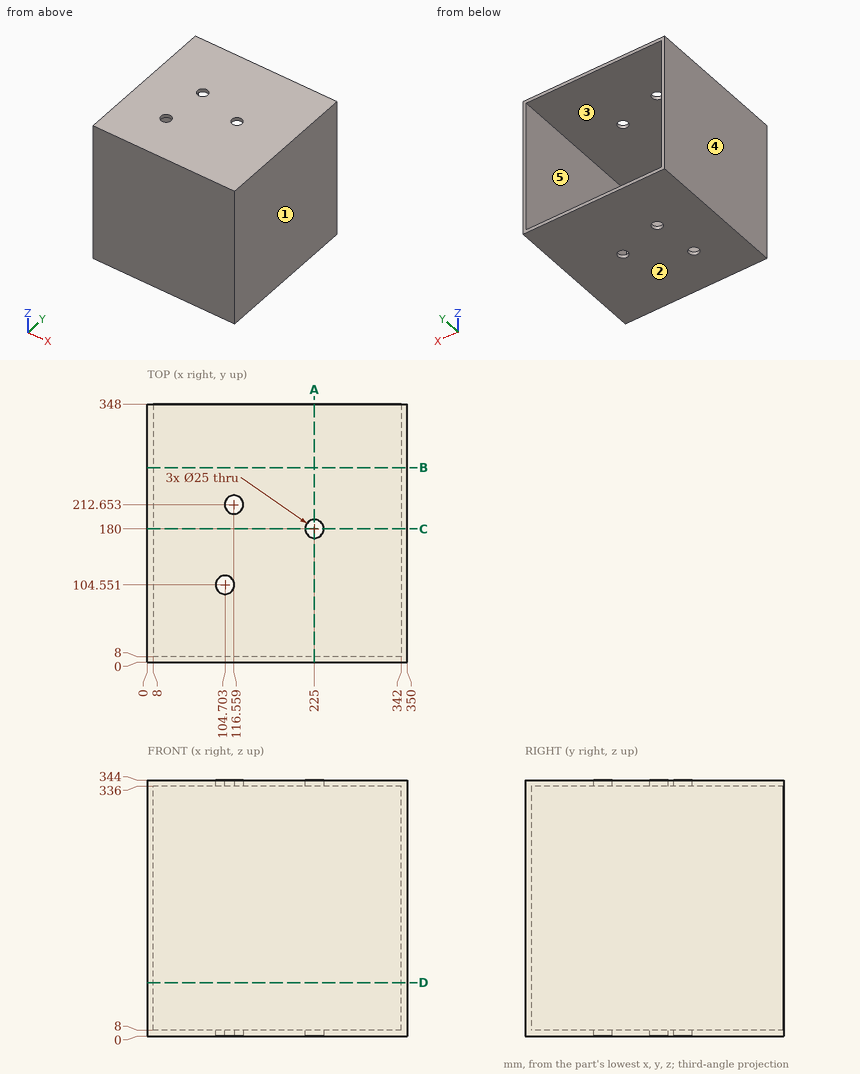
Verification items for this drawing (mm, ordinates from the low corner). A direction names the side the tool comes from. Round coordinates to 2 decimals unless told otherwise and drop trailing zeros. Loops run counter-clockwise (first coordinate to the right, second up) from the corner with the lowest first, then second, coordinate; pieces in that order, holes last. Notation, with made-up numbers: (39.5, 63.25) -> (47.5, 63.25) arc R34 ccw to (47.5, 102.25) -> close; hole circle Ø7 at (42, -34.75). An arc over 180 degrees is marked (long way). Write item = value, one per line. Start each with the question number.
1) Sectioned sample at B-B, the plane y = 262.5. Record the cut outline in (x, z), plus the area to 4 significant figures.
2) Set-up check for the marked faces 4 and 5: record each of +Z, -Z, +X, -X, +Y, -Y from which the full face is reachable in a straight line by a thin tool's end or side.
3) Sectioned sample at C-C, the plane y = 180. Record the cut outline in (x, z).
4) Release check for a two-part mould opening along Z. For the marked faces 1, 2 and 3 record: released by +Z, released by -Z, zero draft, split by the parting line, or undercut.
5) Sectioned sample at A-A, the plane x = 225. Record the cut outline in (y, z), plus the area to 3 significant figures.
6) Sectioned sample at D-D, the plane z = 72. Record the cut outline in (x, y), plus the area to 3 significant figures.
7) Thickness scan on probe 1 along X at (y, z) = (307.5, 173); probe 2 along Z at (x, y) = (276, 164); probe 3 along Y at (x, z) = (225, 4.25). Record the ranges inside material, lowest first.
8) Gauge pin test, flat ends, axial feed: pin 1 Ø4 at (x, z) = (117, 42) entering from +Y; pin 2 Ø20 at (x, y) = (104.7, 104.55) entering from +Z. Record the tip position at first contact, or that the pin passes through.
Results are:
q1.outline = (0, 0) -> (350, 0) -> (350, 344) -> (0, 344) -> close; hole (8, 8) -> (342, 8) -> (342, 336) -> (8, 336) -> close
q1.area = 10,850 mm^2
q2.face_4 = +Z, -Z, -X, +Y, -Y
q2.face_5 = +Y
q3.outline = (0, 0) -> (212.5, 0) -> (212.5, 8) -> (8, 8) -> (8, 336) -> (212.5, 336) -> (212.5, 344) -> (0, 344) -> close; (237.5, 0) -> (350, 0) -> (350, 344) -> (237.5, 344) -> (237.5, 336) -> (342, 336) -> (342, 8) -> (237.5, 8) -> close
q4.face_1 = zero draft
q4.face_2 = released by -Z
q4.face_3 = undercut
q5.outline = (0, 0) -> (167.5, 0) -> (167.5, 8) -> (8, 8) -> (8, 336) -> (167.5, 336) -> (167.5, 344) -> (0, 344) -> close; (192.5, 0) -> (348, 0) -> (348, 8) -> (192.5, 8) -> close; (192.5, 336) -> (348, 336) -> (348, 344) -> (192.5, 344) -> close
q5.area = 7,790 mm^2
q6.outline = (0, 0) -> (350, 0) -> (350, 348) -> (342, 348) -> (342, 8) -> (8, 8) -> (8, 348) -> (0, 348) -> close
q6.area = 8,240 mm^2
q7.probe_1 = 0 to 8, 342 to 350
q7.probe_2 = 0 to 8, 336 to 344
q7.probe_3 = 0 to 167.5, 192.5 to 348
q8.pin_1 = 8
q8.pin_2 = through
